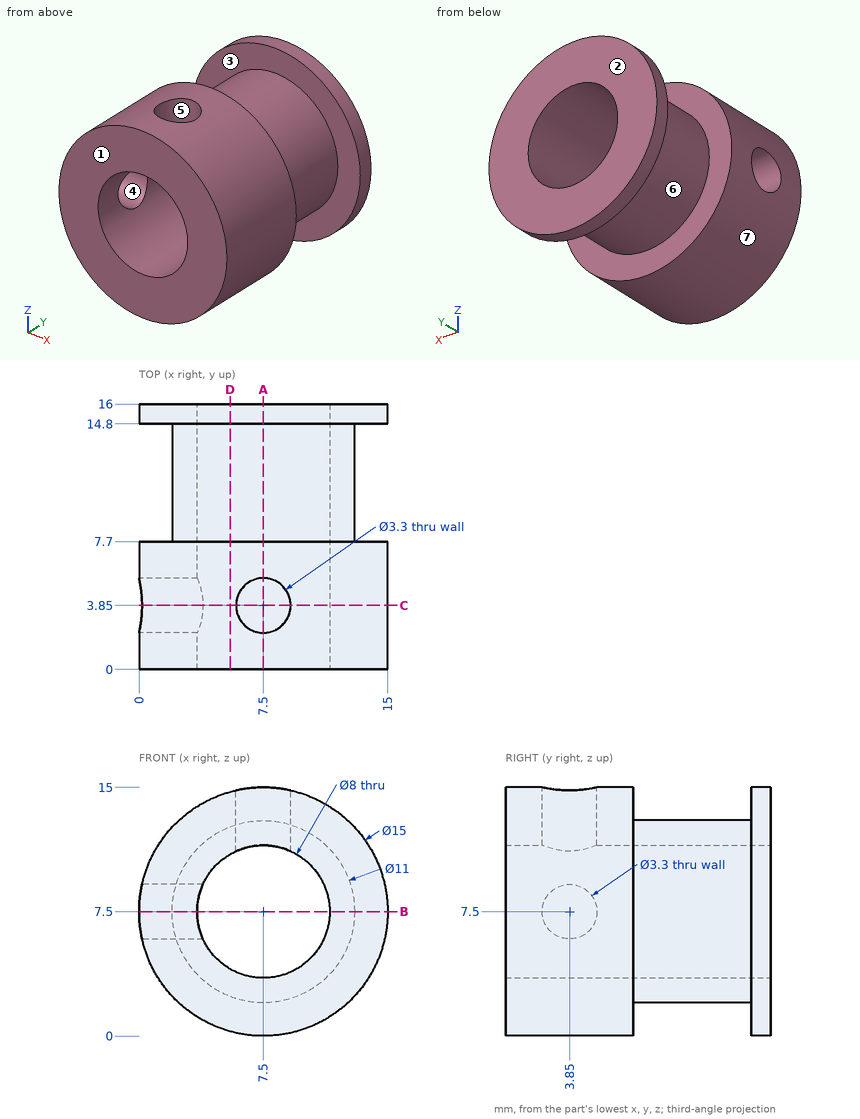
Source: three-view drawing plus pictorial views. Frame: mm from the lowest corner of the part. A direction names the side the tool comes from. Round coordinates to 2 decimals unless told otherwise and drop trailing zeros. Order: outer loops, then holes, each group sorted by start corner. A loop starts at its lowest first (then second) coordinate and runs counter-clockwise, first axis right, second up. Notation, with made-up numbers: (8.5, 52) - (54.5, 52) arc R31 cw to (54.5, 76) - close; hole circle Ø2 at (70, 59). An arc over 180 degrees is marked (long way). Use a Markdown table: item, result.
1. Section B-B on z = 7.5. Return the cut outline in (x, y), then the cut area to 4 significant figures.
Evaluation:
| item | result |
|---|---|
| outline | (0, 0) - (3.5, 0) - (3.5, 2.2) - (0, 2.2) - close; (0, 5.5) - (3.5, 5.5) - (3.5, 16) - (0, 16) - (0, 14.8) - (2, 14.8) - (2, 7.7) - (0, 7.7) - close; (11.5, 0) - (15, 0) - (15, 7.7) - (13, 7.7) - (13, 14.8) - (15, 14.8) - (15, 16) - (11.5, 16) - close |
| area | 72.05 mm^2 |
2. Section C-C on y = 3.85. Return the cut outline in (x, z).
Evaluation:
| item | result |
|---|---|
| outline | (0.18, 5.85) arc R7.5 ccw (long way) to (9.15, 14.82) - (9.15, 11.14) arc R4 cw (long way) to (3.86, 5.85) - close; (0.18, 9.15) - (3.86, 9.15) arc R4 cw to (5.85, 11.14) - (5.85, 14.82) arc R7.5 ccw to start |
3. First-contact query: pin 1 (2 mm diameter, centred on x = 12, y = 2.5, fed in from -Z); pin 2 (3 mm diameter, centred on y = 7, z = 4.5, fed in from +X); pin 3 (8 mm diameter, centred on y = 8.5, z = 2.5, fed in from +X). Flat tips, straight axial feed; report the tip coordinate or a pass-through.
Evaluation:
| item | result |
|---|---|
| pin 1 | z = 0.87 |
| pin 2 | x = 14.85 |
| pin 3 | x = 14.92 |
4. Material intervals for probe 1 along Z at (x, y) = (7.5, 7.5); probe 2 along Z at (x, y) = (7.5, 8); probe 3 along Y at (x, z) = (8.25, 13.5), sorted ascending.
Evaluation:
| item | result |
|---|---|
| probe 1 | 0 to 3.5, 11.5 to 15 |
| probe 2 | 2 to 3.5, 11.5 to 13 |
| probe 3 | 0 to 2.38, 5.32 to 7.7, 14.8 to 16 |
5. Mould query, pull axis Y, two halves, no side actions, for the marked faces 1, 2 and 3. Classes: +Y half, -Y half, draft (parallel to the pull), parting line (faces both ways), or undercut.
Evaluation:
| item | result |
|---|---|
| face 1 | -Y half |
| face 2 | +Y half |
| face 3 | undercut |
6. Access query for the marked faces 4, 5, 6 and 7. Directions: +Z, -Z, +X, -X, +Y, -Y. A direction counts if a zero-diameter tool reaches every point of the face in a straight line with its end or side. Return the directions, or none.
Evaluation:
| item | result |
|---|---|
| face 4 | -X |
| face 5 | +Z |
| face 6 | none |
| face 7 | +Y, -Y |
7. Section D-D on x = 5.5. Return the cut outline in (y, z), then the cut area to 3 significant figures.
Evaluation:
| item | result |
|---|---|
| outline | (0, 0.27) - (7.7, 0.27) - (7.7, 2.38) - (14.8, 2.38) - (14.8, 0.27) - (16, 0.27) - (16, 4.04) - (0, 4.04) - close; (0, 10.96) - (16, 10.96) - (16, 14.73) - (14.8, 14.73) - (14.8, 12.62) - (7.7, 12.62) - (7.7, 14.73) - (0, 14.73) - close |
| area | 90.6 mm^2 |
8. Section A-A on x = 7.5. Return the cut outline in (y, z).
Evaluation:
| item | result |
|---|---|
| outline | (0, 0) - (7.7, 0) - (7.7, 2) - (14.8, 2) - (14.8, 0) - (16, 0) - (16, 3.5) - (0, 3.5) - close; (0, 11.5) - (2.2, 11.5) - (2.2, 15) - (0, 15) - close; (5.5, 11.5) - (16, 11.5) - (16, 15) - (14.8, 15) - (14.8, 13) - (7.7, 13) - (7.7, 15) - (5.5, 15) - close |
